Read the model definition and answer for the solid it produces. Units are mm, in the model's axes. Round coordinates to 2 decimals unless told otherwise and drop trailing zeros. Order: outer loops, then holes, each group sorted by start corner. A loop starts at its lowest first (then second) coordinate and runs counter-clockwise, first axis right, second up. Notation, with made-up numbers: (-32.75, 30.5) -> (16.25, 30.5) arc R14 ccw to (16.25, 54.5) -> close; hole circle Ø3 at (26, -13). An arc over 180 degrees is marked (long way). Use a Markdown table: item, result. Add a question column.
1. Section B-B, the plane y = -3.5 is taken. Give the vertices of the cut face in (x, z).
2. Section A-A, the plane y = -17.5 is taken. Give the vertices of the cut face in (x, z).
3. Given pin 1 (2 mm diameter, centred on y = -16.5, z = 6.5, fed in from -X); pin 2 (0.6 mm diameter, centred on x = 0.5, z = 9.5, fed in from -Y); pin 3 (6 mm diameter, centred on x = -4, y = -8, fed in from -Z); pin 4 (5 mm diameter, centred on x = -1, z = 6.5, fed in from -Y), each flat-ended and moving along its own axis, determine where each tip first touches the part or whether it passes through.
4. Consider L1, parallel to Y at x = -1.5, z = 19.5; L2, parallel to Y at x = 2.75, z = 14.75; L3, parallel to Z at x = -6, y = -7.25. Determine where each line is inside the solid, lowest interval first. Write a range as [from, to].
```python
from build123d import *

# Parameters (mm, degrees)
F0_R      = 10
F1_DEPTH  = 1
F2_R      = 9.5
F3_DEPTH  = 1
F4_R      = 9
F5_DEPTH  = 1
F6_R      = 8.5
F7_DEPTH  = 1
F8_R      = 8
F9_DEPTH  = 1
F10_R     = 7.5
F11_DEPTH = 1
F12_R     = 7
F13_DEPTH = 1
F14_R     = 6.5
F15_DEPTH = 1
F16_R     = 6
F17_DEPTH = 1
F18_R     = 5.5
F19_DEPTH = 1
F20_R     = 5
F21_DEPTH = 1
F22_R     = 4.5
F23_DEPTH = 1
F24_R     = 4
F25_DEPTH = 1
F26_R     = 3.5
F27_DEPTH = 1
F28_R     = 3
F29_DEPTH = 1
F30_R     = 2.5
F31_DEPTH = 1
F32_R     = 2
F33_DEPTH = 1
F34_R     = 1.5
F35_DEPTH = 1
F36_R     = 1
F37_DEPTH = 1
F38_R     = 0.5
F39_DEPTH = 1


with BuildPart() as f1:
    # F0 (on Front) → F1 (new body)
    with BuildSketch(Plane.XZ):
        with Locations((0, 10.208829)):
            Circle(F0_R)
    extrude(amount=F1_DEPTH)

    # F2 (on face) → F3 (join)
    with BuildSketch(Plane.XZ.offset(1)):
        with Locations((0, 10.208829)):
            Circle(F2_R)
    extrude(amount=F3_DEPTH)

    # F4 (on face) → F5 (join)
    with BuildSketch(Plane.XZ.offset(2)):
        with Locations((0, 10.208829)):
            Circle(F4_R)
    extrude(amount=F5_DEPTH)

    # F6 (on face) → F7 (join)
    with BuildSketch(Plane.XZ.offset(3)):
        with Locations((0, 10.208829)):
            Circle(F6_R)
    extrude(amount=F7_DEPTH)

    # F8 (on face) → F9 (join)
    with BuildSketch(Plane.XZ.offset(4)):
        with Locations((0, 10.208829)):
            Circle(F8_R)
    extrude(amount=F9_DEPTH)

    # F10 (on face) → F11 (join)
    with BuildSketch(Plane.XZ.offset(5)):
        with Locations((0, 10.208829)):
            Circle(F10_R)
    extrude(amount=F11_DEPTH)

    # F12 (on face) → F13 (join)
    with BuildSketch(Plane.XZ.offset(6)):
        with Locations((0, 10.208829)):
            Circle(F12_R)
    extrude(amount=F13_DEPTH)

    # F14 (on face) → F15 (join)
    with BuildSketch(Plane.XZ.offset(7)):
        with Locations((0, 10.208829)):
            Circle(F14_R)
    extrude(amount=F15_DEPTH)

    # F16 (on face) → F17 (join)
    with BuildSketch(Plane.XZ.offset(8)):
        with Locations((0, 10.208829)):
            Circle(F16_R)
    extrude(amount=F17_DEPTH)

    # F18 (on face) → F19 (join)
    with BuildSketch(Plane.XZ.offset(9)):
        with Locations((0, 10.208829)):
            Circle(F18_R)
    extrude(amount=F19_DEPTH)

    # F20 (on face) → F21 (join)
    with BuildSketch(Plane.XZ.offset(10)):
        with Locations((0, 10.208829)):
            Circle(F20_R)
    extrude(amount=F21_DEPTH)

    # F22 (on face) → F23 (join)
    with BuildSketch(Plane.XZ.offset(11)):
        with Locations((0, 10.208829)):
            Circle(F22_R)
    extrude(amount=F23_DEPTH)

    # F24 (on face) → F25 (join)
    with BuildSketch(Plane.XZ.offset(12)):
        with Locations((0, 10.208829)):
            Circle(F24_R)
    extrude(amount=F25_DEPTH)

    # F26 (on face) → F27 (join)
    with BuildSketch(Plane.XZ.offset(13)):
        with Locations((0, 10.208829)):
            Circle(F26_R)
    extrude(amount=F27_DEPTH)

    # F28 (on face) → F29 (join)
    with BuildSketch(Plane.XZ.offset(14)):
        with Locations((0, 10.208829)):
            Circle(F28_R)
    extrude(amount=F29_DEPTH)

    # F30 (on face) → F31 (join)
    with BuildSketch(Plane.XZ.offset(15)):
        with Locations((0, 10.208829)):
            Circle(F30_R)
    extrude(amount=F31_DEPTH)

    # F32 (on face) → F33 (join)
    with BuildSketch(Plane.XZ.offset(16)):
        with Locations((0, 10.208829)):
            Circle(F32_R)
    extrude(amount=F33_DEPTH)

    # F34 (on face) → F35 (join)
    with BuildSketch(Plane.XZ.offset(17)):
        with Locations((0, 10.208829)):
            Circle(F34_R)
    extrude(amount=F35_DEPTH)

    # F36 (on face) → F37 (join)
    with BuildSketch(Plane.XZ.offset(18)):
        with Locations((0, 10.208829)):
            Circle(F36_R)
    extrude(amount=F37_DEPTH)

    # F38 (on face) → F39 (join)
    with BuildSketch(Plane.XZ.offset(19)):
        with Locations((0, 10.208829)):
            Circle(F38_R)
    extrude(amount=F39_DEPTH)


solid = f1.part
```
Verdict:
| question | item | result |
|---|---|---|
| 1 | outline | circle Ø17 at (0, 10.21) |
| 2 | outline | circle Ø3 at (0, 10.21) |
| 3 | pin 1 | passes through |
| 3 | pin 2 | stops at y = -19 |
| 3 | pin 3 | stops at z = 2.92 |
| 3 | pin 4 | stops at y = -18 |
| 4 | L1 | y = [-2, 0] |
| 4 | L2 | y = [-10, 0] |
| 4 | L3 | z = [7.71, 12.71] |
